```python
from build123d import *

# Parameters (mm, degrees)
BOSS_EXTRUDE1_DEPTH          = 609.6
F_5_16_18_TAPPED_HOLE1_D     = 6.5278
F_5_16_18_TAPPED_HOLE1_DEPTH = 4.7625


with BuildPart() as part:
    # Sketch1 → Boss-Extrude1 (new body, symmetric)
    with BuildSketch(Plane.XY):
        with BuildLine():
            Line((-20.6375, 38.1), (20.6375, 38.1))
            ThreePointArc((20.6375, 38.1), (24.005096045, 36.705096045), (25.4, 33.3375))
            Line((25.4, 33.3375), (25.4, -33.3375))
            ThreePointArc((25.4, -33.3375), (24.005096045, -36.705096045), (20.6375, -38.1))
            Line((20.6375, -38.1), (-20.6375, -38.1))
            ThreePointArc((-20.6375, -38.1), (-24.005096045, -36.705096045), (-25.4, -33.3375))
            Line((-25.4, -33.3375), (-25.4, 33.3375))
            ThreePointArc((-25.4, 33.3375), (-24.005096045, 36.705096045), (-20.6375, 38.1))
        make_face()
        with BuildLine():
            Line((-19.05, 33.3375), (19.05, 33.3375))
            ThreePointArc((19.05, 33.3375), (20.172532015, 32.872532015), (20.6375, 31.75))
            Line((20.6375, 31.75), (20.6375, -31.75))
            ThreePointArc((20.6375, -31.75), (20.172532015, -32.872532015), (19.05, -33.3375))
            Line((19.05, -33.3375), (-19.05, -33.3375))
            ThreePointArc((-19.05, -33.3375), (-20.172532015, -32.872532015), (-20.6375, -31.75))
            Line((-20.6375, -31.75), (-20.6375, 31.75))
            ThreePointArc((-20.6375, 31.75), (-20.172532015, 32.872532015), (-19.05, 33.3375))
        make_face(mode=Mode.SUBTRACT)
    extrude(amount=BOSS_EXTRUDE1_DEPTH, both=True)

    # 5/16-18 Tapped Hole1
    with Locations(Plane(origin=(0, 38.1, 0), x_dir=(1, 0, 0), z_dir=(0, 1, 0))):
        with Locations((-12.7, -508), (-12.7, 25.4)):
            Hole(F_5_16_18_TAPPED_HOLE1_D / 2, depth=F_5_16_18_TAPPED_HOLE1_DEPTH)


solid = part.part
```
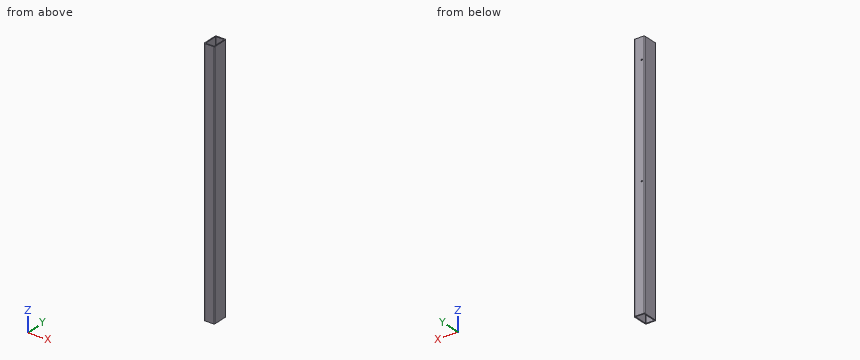
Input: part model. Units: mm. Frame: model coordinates. Coordinates: 2 decimals unless noted, no trailing zeros. Write each loop counter-clockwise with the first axis right and the second up, starting at its lowest first coordinate (ties: lowest second). Pieces come first, ordered by that corner, then holes.
1) Material intervals for line 1 along Z through (x, y) = (-12.7, 36.9); line 2 along Z through (x, y) = (-12, 36); line 3 along Y through (x, z) = (-18.5, 446), sorted ascending.
2) Section C-C on y = 9.5. Output: boundary loops of the cut face in (x, z), and give its area (3 significant figures).
3) Section B-B on x = 10. Output: boundary loops of the cut face in (y, z), and give its area (3 significant figures).
Check result:
1. line 1: z = -609.6 to -28.66, -22.14 to 504.74, 511.26 to 609.6
1. line 2: z = -609.6 to -28.59, -22.21 to 504.81, 511.19 to 609.6
1. line 3: y = -38.1 to -33.34, 33.34 to 38.1
2. outline: (-25.4, -609.6) - (-20.64, -609.6) - (-20.64, 609.6) - (-25.4, 609.6) - close; (20.64, -609.6) - (25.4, -609.6) - (25.4, 609.6) - (20.64, 609.6) - close
2. area: 11,600 mm2
3. outline: (-38.1, -609.6) - (-33.34, -609.6) - (-33.34, 609.6) - (-38.1, 609.6) - close; (33.34, -609.6) - (38.1, -609.6) - (38.1, 609.6) - (33.34, 609.6) - close
3. area: 11,600 mm2
